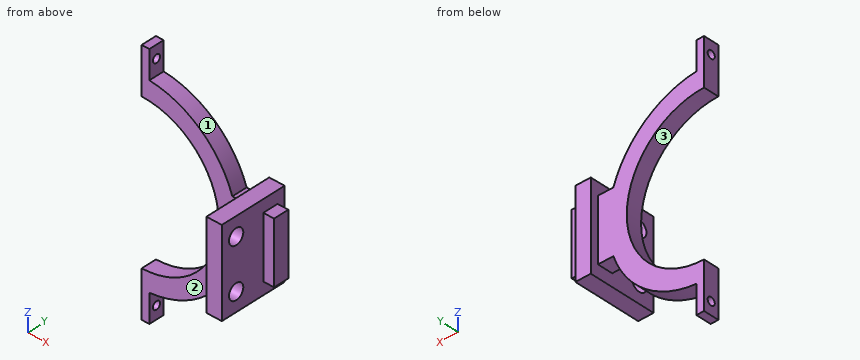
from build123d import *

# Parameters (mm, degrees)
BOSS_EXTRUDE1_DEPTH = 5
SKETCH4_W           = 28
SKETCH4_H           = 22
SKETCH4_R           = 2.5
BOSS_EXTRUDE3_DEPTH = 5
SKETCH6_W           = 20
SKETCH6_H           = 5
BOSS_EXTRUDE4_DEPTH = 3.5
SKETCH8_R           = 1.25
CUT_EXTRUDE1_DEPTH  = 3.5


with BuildPart() as part:
    # Sketch1 → Boss-Extrude1 (new body)
    with BuildSketch(Plane(origin=(0, 0, 0), x_dir=(1, 0, 0), z_dir=(0, 1, 0))):
        with BuildLine():
            Line((0, -25), (0, -40))
            Line((0, -40), (2.5, -40))
            Line((2.5, -40), (2.5, -30.899029111))
            ThreePointArc((2.5, -30.899029111), (19.044247329, -24.460511926), (29.342801502, -10))
            Line((29.342801502, -10), (39.342801502, -10))
            Line((39.342801502, -10), (39.342801502, 10))
            Line((39.342801502, 10), (29.342801502, 10))
            ThreePointArc((29.342801502, 10), (19.044247329, 24.460511926), (2.5, 30.899029111))
            Line((2.5, 30.899029111), (2.5, 40))
            Line((2.5, 40), (0, 40))
            Line((0, 40), (0, 25))
            ThreePointArc((0, 25), (25, 0), (0, -25))
        make_face()
    extrude(amount=BOSS_EXTRUDE1_DEPTH)

    # Sketch4 → Boss-Extrude3 (add)
    with BuildSketch(Plane(origin=(39.342801502, 0, 0), x_dir=(0, 0, -1), z_dir=(1, 0, 0))):
        with Locations((0, -3.5)):
            Rectangle(SKETCH4_W, SKETCH4_H)
        with Locations((8, -9.5)):
            Circle(SKETCH4_R, mode=Mode.SUBTRACT)
        with Locations((-8, -9.5)):
            Circle(SKETCH4_R, mode=Mode.SUBTRACT)
    extrude(amount=-BOSS_EXTRUDE3_DEPTH)

    # Sketch6 → Boss-Extrude4 (add)
    with BuildSketch(Plane(origin=(39.342801502, 0, 0), x_dir=(0, 0, -1), z_dir=(1, 0, 0))):
        with Locations((0, 2.5)):
            Rectangle(SKETCH6_W, SKETCH6_H)
    extrude(amount=BOSS_EXTRUDE4_DEPTH)

    # Sketch8 → Cut-Extrude1 (cut, through all)
    with BuildSketch(Plane(origin=(2.5, 0, 0), x_dir=(0, 0, -1), z_dir=(1, 0, 0))):
        with Locations((-35.899029111, 2.5)):
            Circle(SKETCH8_R)
        with Locations((35.899029111, 2.5)):
            Circle(SKETCH8_R)
    extrude(amount=-CUT_EXTRUDE1_DEPTH, mode=Mode.SUBTRACT)


solid = part.part
Here's how the part is built. I have some questions about the finished solid (model axes, mm). Face numbers are marked on the shaded views. Coordinates: 2 decimals unless noted, no trailing zeros. Loops run counter-clockwise (first coordinate to the right, second up) from the corner with the lowest first, then second, coordinate; pieces in that order, holes last.
1. Imagine slicing it at A-A, the plane y = -9.5. Please give me the cut outline in (x, z).
2. I need wall thicknesses on L1, parallel to Y at x = 38, z = -8; L2, parallel to X at y = -9.25, z = 1.5; L3, parallel to Z at x = 30, y = 4.75. Which ranges of each line are inside material? Lowest first, please.
3. Imagine slicing it at D-D, the plane x = 17.5. Please give me the cut outline in (y, z).
4. If we mould it in two halves opening along Z, with no side actions, what happens to the marked faces 1, 2 and 3? For each: pulls with the +Z half, pulls with the -Z half, needs draft (parallel to the pull), parting line crosses it, or undercut.
5. Imagine slicing it at C-C, the plane z = -8. Please give me the cut outline in (x, y).
6. For P1, Ø10, axis at x = 22.5, z = -30.5, coming from the -Y side; P2, Ø10.5, axis at x = 19.5, z = -10, coming from the -Y side; P3, Ø4, axis at x = 41, y = 3.5, coming from the +Z side; P4, Ø5.5, axis at y = 3, z = -35.5, coming from the +X side, each with a flat end and sliding along its axis, tell me the tip position at first contact or that it passes through.
7. Imagine slicing it at B-B, the plane z = 0. Please give me the cut outline in (x, y).
Taken from the geometry:
1. outline: (34.34, -14) - (39.34, -14) - (39.34, -10.5) - (34.34, -10.5) - close; (34.34, -5.5) - (39.34, -5.5) - (39.34, 5.5) - (34.34, 5.5) - close; (34.34, 10.5) - (39.34, 10.5) - (39.34, 14) - (34.34, 14) - close
2. L1: y = -14.5 to -12, -7 to 7.5
2. L2: x = 34.34 to 39.34
2. L3: z = -10 to 10
3. outline: (0, -25.59) - (5, -25.59) - (5, -17.85) - (0, -17.85) - close; (0, 17.85) - (5, 17.85) - (5, 25.59) - (0, 25.59) - close
4. face 1: pulls with the +Z half
4. face 2: needs draft
4. face 3: undercut
5. outline: (23.69, 0) - (34.34, 0) - (34.34, -7) - (39.34, -7) - (39.34, 0) - (42.84, 0) - (42.84, 5) - (39.34, 5) - (39.34, 7.5) - (34.34, 7.5) - (34.34, 5) - (23.69, 5) - close; (34.34, -14.5) - (39.34, -14.5) - (39.34, -12) - (34.34, -12) - close
6. P1: passes through
6. P2: stops at y = 0
6. P3: stops at z = 14
6. P4: stops at x = 2.5
7. outline: (25, 0) - (34.34, 0) - (34.34, -14.5) - (39.34, -14.5) - (39.34, 0) - (42.84, 0) - (42.84, 5) - (39.34, 5) - (39.34, 7.5) - (34.34, 7.5) - (34.34, 5) - (25, 5) - close
